The listing builds one solid part. Answer for the finished solid, in the listing's coordinates (mm). A direction names the side the tool comes from. Round coordinates to 2 decimals unless told otherwise and drop trailing zeros. Write each loop counter-clockwise with the first axis right and the second up, starting at its lowest first coordinate (ties: lowest second). Pieces come first, ordered by that corner, then holes.
(1) A cutting plane is placed at B-B, the plane z = 0. Give the vertices of the cut face in (x, y), and give its area (3 significant figures).
(2) Find the intervals of material crossed by probe 1 along X at (y, z) = (24.25, 9.45); probe 2 along Z at (x, y) = (3.25, 15.5); probe 3 along Y at (x, z) = (-1, -7), in increasing order.
(3) For faces 4 (the face through (-0.26, 22.267, -9.493)), 5 (the face through (5, 12, 0)), 6 (the face through (-4.88, 3.45, 1.08)), 7 (the face through (0, 19, 9)), determine the directions among +Z, -Z, +X, -X, +Y, -Y from which every point of the face is accessible in a straight line to the end or side of a thin tool.
(4) The mould has two halves that part along Z. Classify faces 1 (the face through (-2.221, 26.357, 10.014)), 2 (the face through (0, 19, 11)), 3 (the face through (0, 19, -9)): +Z half, -Z half, draft (parallel to the pull), parting line (faces both ways), or undercut.
(5) A cutting plane is placed at D-D, the plane y = 11.5. Give the vertices of the cut face in (x, z).
(6) A cutting plane is placed at A-A, the plane y = 15.5. Give the vertices of the cut face in (x, z).
(7) Each of these flat-tipped pins is pushed along its axis until it touches: pin 1 Ø6.5 at (x, z) = (-2, 4) entering from +Y; pin 2 Ø1.5 at (y, z) = (14.5, 3) entering from -X; pin 3 Ø0.6 at (x, z) = (5, -1) entering from +Y. Where does it stop, or does it pass through?
(8) A cutting plane is placed at C-C, the plane y = 24.25. Give the vertices of the cut face in (x, z).
from build123d import *

# Parameters (mm, degrees)
SKETCH1_R                = 7.5
BOSS_EXTRUDE1_DEPTH      = 10
SKETCH5_R                = 6
BOSS_EXTRUDE2_DEPTH      = 2
FILLET2_R                = 1
BOSS_EXTRUDE3_DEPTH      = 6
BOSS_EXTRUDE3_DEPTH_BACK = 6
CUT_EXTRUDE4_DEPTH       = 29
CUT_EXTRUDE5_DEPTH       = 19
CUT_EXTRUDE5_DEPTH_BACK  = 1
SKETCH10_R               = 2
SKETCH12_R               = 5
CUT_EXTRUDE6_DEPTH       = 7
CUT_EXTRUDE7_START       = -36
CUT_EXTRUDE7_DEPTH       = 36


with BuildPart() as part:
    # Sketch1 → Boss-Extrude1 (new body)
    with BuildSketch(Plane(origin=(0, 0, 0), x_dir=(1, 0, 0), z_dir=(0, 1, 0))):
        with Locations(Location((0, 0, 0), (0, 0, 270))):
            Circle(SKETCH1_R)
    extrude(amount=BOSS_EXTRUDE1_DEPTH)

    # Sketch5 → Boss-Extrude2 (add)
    with BuildSketch(Plane(origin=(0, 10, 0), x_dir=(1, 0, 0), z_dir=(0, 1, 0))):
        with Locations(Location((0, 0, 0), (0, 0, 270))):
            Circle(SKETCH5_R)
    extrude(amount=BOSS_EXTRUDE2_DEPTH)

    # Fillet2
    fillet2_edges = [part.edges().sort_by_distance(p)[0] for p in [
        (0, 10, -6),
    ]]
    fillet(fillet2_edges, radius=FILLET2_R)

    # Sketch6 → Boss-Extrude3 (add, two sides: drawn at the far end of the back side and taken through both)
    with BuildSketch(Plane(origin=(0, 0, 0), x_dir=(0, 0, -1), z_dir=(1, 0, 0)).offset(-BOSS_EXTRUDE3_DEPTH_BACK)):
        Polygon((6, 12), (-6, 12), (-11, 12), (-11, 27), (-9, 27), (-9, 14), (9, 14), (9, 27), (11, 27), (11, 12), align=None)
    extrude(amount=BOSS_EXTRUDE3_DEPTH + BOSS_EXTRUDE3_DEPTH_BACK)

    # Sketch9 → Cut-Extrude4 (cut)
    with BuildSketch(Plane.XY.offset(11)):
        with BuildLine():
            Line((-6, 27), (-6, 21))
            ThreePointArc((-6, 21), (-4.052343178, 25.052343178), (0, 27))
            Line((0, 27), (-6, 27))
        make_face()
        with BuildLine():
            ThreePointArc((0, 27), (4.052343178, 25.052343178), (6, 21))
            Line((6, 21), (6, 27))
            Line((6, 27), (0, 27))
        make_face()
    extrude(amount=-CUT_EXTRUDE4_DEPTH, mode=Mode.SUBTRACT)

    # Sketch10 → Cut-Extrude5 (cut, two sides: drawn at the far end of the back side and taken through both)
    with BuildSketch(Plane(origin=(0, 0, 9), x_dir=(-1, 0, 0), z_dir=(0, 0, -1)).offset(-CUT_EXTRUDE5_DEPTH_BACK)):
        with Locations(Location((0, 24.25, 0), (0, 0, 180))):
            Circle(SKETCH10_R)
    extrude(amount=CUT_EXTRUDE5_DEPTH + CUT_EXTRUDE5_DEPTH_BACK, mode=Mode.SUBTRACT)

    # Sketch12 → Cut-Extrude6 (cut)
    with BuildSketch(Plane.XZ):
        with Locations(Location((0, 0, 0), (0, 0, 270))):
            Circle(SKETCH12_R)
    extrude(amount=-CUT_EXTRUDE6_DEPTH, mode=Mode.SUBTRACT)

    # Sketch13 → Cut-Extrude7 (cut)
    with BuildSketch(Plane(origin=(0, 0, -11), x_dir=(-1, 0, 0), z_dir=(0, 0, -1)).offset(CUT_EXTRUDE7_START)):
        with BuildLine():
            Line((-4.052343178, 12), (-4.052343178, 25.052343178))
            ThreePointArc((-4.052343178, 25.052343178), (-5.371235948, 23.192018094), (-6, 21))
            Line((-6, 21), (-6, 12))
            Line((-6, 12), (-4.052343178, 12))
        make_face()
        with BuildLine():
            Line((4.052343178, 25.052343178), (4.052343178, 12))
            Line((4.052343178, 12), (6, 12))
            Line((6, 12), (6, 21))
            ThreePointArc((6, 21), (5.371235948, 23.192018094), (4.052343178, 25.052343178))
        make_face()
    extrude(amount=CUT_EXTRUDE7_DEPTH, mode=Mode.SUBTRACT)


solid = part.part
Solutions:
1. outline: (-7.5, 0) - (-5, 0) - (-5, 7) - (5, 7) - (5, 0) - (7.5, 0) - (7.5, 10) - (7, 10) arc R1 cw to (6, 11) - (6, 12) - (4.05, 12) - (4.05, 14) - (-4.05, 14) - (-4.05, 12) - (-6, 12) - (-6, 11) arc R1 cw to (-7, 10) - (-7.5, 10) - close
1. area: 121 mm2
2. probe 1: x = -4.05 to -2, 2 to 4.05
2. probe 2: z = -11 to -9, 9 to 11
2. probe 3: y = 0 to 10, 12 to 14
3. face 4: none
3. face 5: +Z, -Z, +X, +Y
3. face 6: -Y
3. face 7: +X, -X, +Y
4. face 1: draft
4. face 2: +Z half
4. face 3: undercut
5. outline: circle Ø12 at (0, 0)
6. outline: (-4.05, -11) - (4.05, -11) - (4.05, -9) - (-4.05, -9) - close; (-4.05, 9) - (4.05, 9) - (4.05, 11) - (-4.05, 11) - close
7. pin 1: stops at y = 14
7. pin 2: stops at x = -4.05
7. pin 3: stops at y = 12
8. outline: (-4.05, -11) - (4.05, -11) - (4.05, -9) - (2, -9) - (2, -10) - (-2, -10) - (-2, -9) - (-4.05, -9) - close; (-4.05, 9) - (-2, 9) - (-2, 10) - (2, 10) - (2, 9) - (4.05, 9) - (4.05, 11) - (-4.05, 11) - close
